Input: part model. Units: mm. Frame: model coordinates. A direction names the side the tool comes from. Give positions to 0.01 mm unless a question says otherwise; leave off trailing zeros. Loops run counter-clockwise (first coordinate to the right, second up) from the corner with the lowest first, then second, coordinate; pieces in that order, holes last. Notation, with made-up numbers: M 4,-9 L 45,-9 A25 ccw 45,13 Z; hole C 31.25,44.25 d5. An arc over 180 degrees is marked long. Answer as a JSON object with one key per item and string values. Group by question number.
1) Draft query along Y for faces 1 (the flat face through (-9, 5, 3)), 2 (the flat face through (10, 0, 3)), 3 (the flat face through (0, -5, 3)). Return one class per face: +Y half, -Y half, draft (parallel to the pull), parting line (faces both ways), or undercut.
2) Ray query, L1, parallel to X at y = -1.5, z = 3.7; L2, parallel to Y at x = 0, z = 0.85; L3, parallel to Y at x = 9, z = 0.65. Return the intervals inside material, ascending.
3) Section query C-C on x = -4.25. Return loops of the section in (y, z).
4) Access query for faces 4 (the flat face through (-10, 0, 3)), 5 (the flat face through (0, 14, 0)). Directions: +Z, -Z, +X, -X, +Y, -Y. A direction counts if a zero-diameter tool reaches every point of the face in a straight line with its end or side. Return the directions, or none.
5) Section query B-B on y = 9. Return loops of the section in (x, z).
6) Section query A-A on z = 1.15. Return loops of the section in (x, y).
7) First-contact query: P1, Ø8, axis at x = -7, y = 22.5, coming from the -Z side; P2, Ø2, axis at x = 8.5, z = 2, coming from the +Y side; P3, Ø2, axis at x = -9, z = 4.5, coming from the +Y side; P4, Ø3, axis at y = 25.5, z = 2.5, coming from the +X side. Flat tips, straight axial feed; report the tip coordinate or a pass-through.
from build123d import *

# Parameters (mm, degrees)
ESQUISSE1_W        = 20
ESQUISSE1_H        = 10
BOSS_EXTRU_1_DEPTH = 6
ESQUISSE2_R        = 15
BOSS_EXTRU_2_DEPTH = 6


with BuildPart() as part:
    # Esquisse1 → Boss.-Extru.1 (new body)
    with BuildSketch(Plane.XY):
        Rectangle(ESQUISSE1_W, ESQUISSE1_H)
    extrude(amount=BOSS_EXTRU_1_DEPTH)

    # Esquisse2 → Boss.-Extru.2 (add)
    with BuildSketch(Plane.XY.offset(6)):
        with Locations((0, 18)):
            Circle(ESQUISSE2_R)
    extrude(amount=-BOSS_EXTRU_2_DEPTH)


solid = part.part
Output:
{
 "1": {"face 1": "undercut", "face 2": "draft", "face 3": "-Y half"},
 "2": {"L1": "x = -10 to 10", "L2": "y = -5 to 33", "L3": "y = -5 to 5, 6 to 30"},
 "3": {"outline": "M -5,0 L 32.39,0 L 32.39,6 L -5,6 Z"},
 "4": {"face 4": "+Z, -Z, -X, -Y", "face 5": "-Z, +X, -X, +Y, -Y"},
 "5": {"outline": "M -12,0 L 12,0 L 12,6 L -12,6 Z"},
 "6": {"outline": "M -10,-5 L 10,-5 L 10,5 L 7.48,5 A15 ccw long -7.48,5 L -10,5 Z"},
 "7": {"P1": "stops at z = 0", "P2": "stops at y = 30.99", "P3": "stops at y = 30.69", "P4": "stops at x = 13.75"}
}
